For this review, take the finished solid that the model builds, in its own axes (mm). Face numbers are marked on the shaded views. Round coordinates to 2 decimals unless told otherwise and drop trailing zeros. Write each loop counter-clockwise with the first axis right and the second up, starting at its lowest first coordinate (ties: lowest second). Pieces come first, ordered by that corner, then holes.
from build123d import *

# Parameters (mm, degrees)
EXTRUDE_1_DEPTH     = 5
SKETCH_3_R          = 4.1
CUT_EXTRUDE_1_DEPTH = 5
SKETCH_5_R          = 3.1
CUT_EXTRUDE_2_DEPTH = 5


with BuildPart() as part:
    # 草图2 → 凸台-拉伸1 (new body)
    with BuildSketch(Plane.XY):
        with BuildLine():
            Line((-30, 30), (30, 30))
            Line((30, 30), (30, 0))
            ThreePointArc((30, 0), (0, -30), (-30, 0))
            Line((-30, 0), (-30, 30))
        make_face()
    extrude(amount=EXTRUDE_1_DEPTH)

    # 草图3 → 切除-拉伸1 (cut)
    with BuildSketch(Plane.XY.offset(5)):
        Circle(SKETCH_3_R)
    extrude(amount=-CUT_EXTRUDE_1_DEPTH, mode=Mode.SUBTRACT)

    # 草图5 → 切除-拉伸2 (cut)
    with BuildSketch(Plane.XY.offset(5)):
        with Locations((0, 25)):
            Circle(SKETCH_5_R)
        with Locations((9.567085809, 23.096988313)):
            Circle(SKETCH_5_R)
        with Locations((17.67766953, 17.67766953)):
            Circle(SKETCH_5_R)
        with Locations((23.096988313, 9.567085809)):
            Circle(SKETCH_5_R)
        with Locations((25, 0)):
            Circle(SKETCH_5_R)
        with Locations((23.096988313, -9.567085809)):
            Circle(SKETCH_5_R)
        with Locations((17.67766953, -17.67766953)):
            Circle(SKETCH_5_R)
        with Locations((9.567085809, -23.096988313)):
            Circle(SKETCH_5_R)
        with Locations((0, -25)):
            Circle(SKETCH_5_R)
        with Locations((-9.567085809, -23.096988313)):
            Circle(SKETCH_5_R)
        with Locations((-17.67766953, -17.67766953)):
            Circle(SKETCH_5_R)
        with Locations((-23.096988313, -9.567085809)):
            Circle(SKETCH_5_R)
        with Locations((-25, 0)):
            Circle(SKETCH_5_R)
        with Locations((-23.096988313, 9.567085809)):
            Circle(SKETCH_5_R)
        with Locations((-17.67766953, 17.67766953)):
            Circle(SKETCH_5_R)
        with Locations((-9.567085809, 23.096988313)):
            Circle(SKETCH_5_R)
    extrude(amount=-CUT_EXTRUDE_2_DEPTH, mode=Mode.SUBTRACT)


solid = part.part
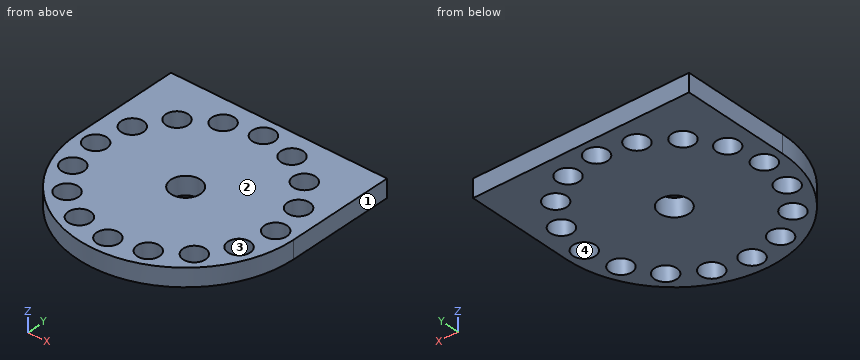
(1) We need section A-A, the plane x = 0. Give the boundary of the cut face in (y, z), and give its area (3 significant figures).
Geometry check:
outline: (-30, 0) - (-28.1, 0) - (-28.1, 5) - (-30, 5) - close; (-21.9, 0) - (-4.1, 0) - (-4.1, 5) - (-21.9, 5) - close; (4.1, 0) - (21.9, 0) - (21.9, 5) - (4.1, 5) - close; (28.1, 0) - (30, 0) - (30, 5) - (28.1, 5) - close
area: 197 mm2
(2) For line 1 along Y through (x, z) = (0, 3.3); line 2 along X through (y, z) = (-1, 2); line 3 along Y through (x, z) = (-11.5, 1.7), list the stretches that pass through material, from the lowest coordinate up.
Geometry check:
line 1: y = -30 to -28.1, -21.9 to -4.1, 4.1 to 21.9, 28.1 to 30
line 2: x = -29.98 to -27.93, -22.07 to -3.98, 3.98 to 22.07, 27.93 to 29.98
line 3: y = -27.71 to -25.52, -20.67 to 20.67, 25.52 to 30
(3) We need section D-D, the plane x = 7.5. Give the boundary of the cut face in (y, z), and give its area (3 significant figures).
Geometry check:
outline: (-29.05, 0) - (-25.41, 0) - (-25.41, 5) - (-29.05, 5) - close; (-20.79, 0) - (20.79, 0) - (20.79, 5) - (-20.79, 5) - close; (25.41, 0) - (30, 0) - (30, 5) - (25.41, 5) - close
area: 249 mm2
(4) We need section B-B, the plane y = 25. Give the boundary of the cut face in (x, z).
Geometry check:
outline: (-30, 0) - (-12.01, 0) - (-12.01, 5) - (-30, 5) - close; (-7.12, 0) - (-3.1, 0) - (-3.1, 5) - (-7.12, 5) - close; (3.1, 0) - (7.12, 0) - (7.12, 5) - (3.1, 5) - close; (12.01, 0) - (30, 0) - (30, 5) - (12.01, 5) - close
(5) For pin 1 Ø1.5 at (x, z) = (-20, 3) entering from -Y, flat-tipped, find the tip position at first contact; note if it passes through.
Geometry check:
pin 1: stops at y = -23.01
(6) Mouldability with a two-part tool opening along X and no side actions: class the marked faces 1, 2, 3 and 4 as pulls with the +X half, pulls with the -X half, needs draft (parallel to the pull), parting line crosses it, or undercut.
Geometry check:
face 1: pulls with the +X half
face 2: needs draft
face 3: undercut
face 4: undercut
(7) We need section C-C, the plane z = 3.7. State how many separate pieces and enclosed holes the cut face has, and give its area (3 significant figures).
Geometry check:
separate pieces: 1
enclosed holes: 17
area: 2,680 mm2
